Source: CAD feature listing. Evaluate the final solid. Frame: model axes, mm. A direction names the side the tool comes from. Round coordinates to 2 decimals unless told otherwise and drop trailing zeros. Write each loop counter-clockwise with the first axis right and the second up, starting at its lowest first coordinate (ties: lowest second). Pieces come first, ordered by that corner, then holes. Notation, with made-up numbers: M 78,80.5 L 121,80.5 A21 ccw 121,90.5 Z; hole C -32.5,4 d6. An arc over 180 degrees is marked long. Use a Markdown table: item, result.
```python
from build123d import *

# Parameters (mm, degrees)
BOSS_EXTRUDE1_OUTLINE_R = 1.75
BOSS_EXTRUDE1_DEPTH     = 4
CUT_EXTRUDE1_DEPTH      = 1


# Read off the part's stored shape, not the designer's step: Boss-Extrude1
with BuildPart() as part:
    # Boss-Extrude1 outline → Boss-Extrude1 (new body)
    with BuildSketch(Plane(origin=(0, 0, 0), x_dir=(1, 0, 0), z_dir=(0, 1, 0))):
        with BuildLine():
            Line((25.196474615, -10.33744254), (36.58307775, -10.33744254))
            ThreePointArc((36.58307775, -10.33744254), (39.019776183, -5.587442326), (41.456474615, -10.33744254))
            Line((41.456474615, -10.33744254), (48.519776182, -10.33744254))
            Line((48.519776182, -10.33744254), (48.519776182, -18.81631662))
            Line((48.519776182, -18.81631662), (58.694776182, -18.81631662))
            Line((58.694776182, -18.81631662), (58.694776182, -4.977921711))
            Line((58.694776182, -4.977921711), (-21.305223818, -4.977921711))
            Line((-21.305223818, -4.977921711), (-21.305223818, -18.81631662))
            Line((-21.305223818, -18.81631662), (-11.130223818, -18.81631662))
            Line((-11.130223818, -18.81631662), (-11.130223818, -10.33744254))
            Line((-11.130223818, -10.33744254), (4.06307775, -10.33744254))
            ThreePointArc((4.06307775, -10.33744254), (6.499776182, -5.587442326), (8.936474615, -10.33744254))
            Line((8.936474615, -10.33744254), (20.32307775, -10.33744254))
            ThreePointArc((20.32307775, -10.33744254), (22.759776182, -5.587442326), (25.196474615, -10.33744254))
        make_face()
        with Locations((-16.305223818, -13.587442433)):
            Circle(BOSS_EXTRUDE1_OUTLINE_R, mode=Mode.SUBTRACT)
        with Locations((53.694776182, -13.587442433)):
            Circle(BOSS_EXTRUDE1_OUTLINE_R, mode=Mode.SUBTRACT)
    extrude(amount=BOSS_EXTRUDE1_DEPTH)

    # Sketch2 → Cut-Extrude1 (cut)
    with BuildSketch(Plane(origin=(0, 4, 0), x_dir=(1, 0, 0), z_dir=(0, 1, 0))):
        Polygon((-16.41198232, -6.812466594), (-14.865187448, -6.812466594), (-14.865187448, -7.382338389), (-15.842110525, -7.382338389), (-15.842110525, -7.992915312), (-14.865187448, -7.992915312), (-14.865187448, -8.562787107), (-15.842110525, -8.562787107), (-15.842110525, -9.987466594), (-16.41198232, -9.987466594), align=None)
        Polygon((-14.417431038, -6.812466594), (-12.382174628, -6.812466594), (-12.382174628, -7.108214791), (-13.782685445, -10.06887685), (-14.287047424, -9.814469799), (-13.117411006, -7.341633261), (-14.417431038, -7.341633261), align=None)
    extrude(amount=-CUT_EXTRUDE1_DEPTH, mode=Mode.SUBTRACT)


solid = part.part
```
Q1. Reachability of faces 4 (the cylindrical face through (6.41, 1.97, 5.59)), 5 (the flat face through (31, 2, 10.337)) from +Z, -Z, +X, -X, +Y, -Y: full face, straight path, thin tool, end or side. Return the list, or none.
Results are:
| item | result |
|---|---|
| face 4 | +Y, -Y |
| face 5 | +Z, +Y, -Y |
Q2. Section A-A on z = 18. Return loops of the section in (x, y).
Results are:
| item | result |
|---|---|
| outline | M -21.31,0 L -11.13,0 L -11.13,4 L -21.31,4 Z; M 48.52,0 L 58.69,0 L 58.69,4 L 48.52,4 Z |
Q3. Line query: L1, parallel to X at y = 1.85, z = 13.5; L2, parallel to X at y = 1.55, z = 17.75. Output: solid intervals per line, ascending.
Results are:
| item | result |
|---|---|
| L1 | -21.31 to -18.05, -14.56 to -11.13, 48.52 to 51.95, 55.44 to 58.69 |
| L2 | -21.31 to -11.13, 48.52 to 58.69 |
Q4. Mould query, pull axis X, two halves, no side actions, for faces 1 (the flat face through (45, 2, 10.337)), 2 (the flat face through (58.695, 2, 12)), 3 (the flat face through (54, 2, 18.816)). Classes: +X half, -X half, draft (parallel to the pull), parting line (faces both ways), or undercut.
Results are:
| item | result |
|---|---|
| face 1 | undercut |
| face 2 | +X half |
| face 3 | draft |
Q5. Section C-C on x = 43. Return loops of the section in (y, z), plus the area to 3 significant figures.
Results are:
| item | result |
|---|---|
| outline | M 0,4.98 L 4,4.98 L 4,10.34 L 0,10.34 Z |
| area | 21.4 mm^2 |
Q6. Section B-B on y = 0.85. Return loops of the section in (x, z), plus the area to 3 significant figures.
Results are:
| item | result |
|---|---|
| outline | M -21.31,4.98 L 58.69,4.98 L 58.69,18.82 L 48.52,18.82 L 48.52,10.34 L 41.46,10.34 A3 cw long 36.58,10.34 L 25.2,10.34 A3 cw long 20.32,10.34 L 8.94,10.34 A3 cw long 4.06,10.34 L -11.13,10.34 L -11.13,18.82 L -21.31,18.82 Z; hole C -16.31,13.59 d3.5; hole C 53.69,13.59 d3.5 |
| area | 510 mm^2 |
